from build123d import *

# Parameters (mm, degrees)
SKETCH1_W           = 38
SKETCH1_H           = 180
BOSS_EXTRUDE1_DEPTH = 25
SKETCH2_W           = 32
SKETCH2_H           = 174
CUT_EXTRUDE1_DEPTH  = 22
CHAMFER1_SIZE       = 10
FILLET1_R           = 5
FILLET2_R           = 2
SKETCH3_W           = 14
SKETCH3_H           = 10
BOSS_EXTRUDE2_DEPTH = 7
SKETCH4_W           = 14
SKETCH4_H           = 10.939467079
BOSS_EXTRUDE3_DEPTH = 7
FILLET3_R           = 3
SKETCH5_W           = 3
SKETCH5_H           = 6
CUT_EXTRUDE2_DEPTH  = 97.958754117
SKETCH6_R           = 3
CUT_EXTRUDE3_DEPTH  = 10


with BuildPart() as part:
    # Sketch1 → Boss-Extrude1 (new body)
    with BuildSketch(Plane(origin=(0, 0, 0), x_dir=(1, 0, 0), z_dir=(0, 1, 0))):
        Rectangle(SKETCH1_W, SKETCH1_H)
    extrude(amount=BOSS_EXTRUDE1_DEPTH)

    # Sketch2 → Cut-Extrude1 (cut)
    with BuildSketch(Plane.XZ):
        Rectangle(SKETCH2_W, SKETCH2_H)
    extrude(amount=-CUT_EXTRUDE1_DEPTH, mode=Mode.SUBTRACT)

    # Chamfer1
    chamfer1_edges = [part.edges().sort_by_distance(p)[0] for p in [
        (-19, 25, 0),
        (16, 22, 0),
        (0, 25, 90),
        (0, 22, -87),
        (-16, 22, 0),
        (0, 22, 87),
        (19, 25, 0),
        (0, 25, -90),
    ]]
    chamfer(chamfer1_edges, length=CHAMFER1_SIZE)

    # Fillet1
    fillet1_edges = [part.edges().sort_by_distance(p)[0] for p in [
        (19, 7.5, 90),
        (-19, 7.5, 90),
        (-19, 7.5, -90),
        (19, 7.5, -90),
    ]]
    fillet(fillet1_edges, radius=FILLET1_R)

    # Fillet2
    fillet2_edges = [part.edges().sort_by_distance(p)[0] for p in [
        (16, 6, -87),
        (-16, 6, -87),
        (-16, 6, 87),
        (16, 6, 87),
    ]]
    fillet(fillet2_edges, radius=FILLET2_R)

    # Sketch3 → Boss-Extrude2 (add)
    with BuildSketch(Plane(origin=(19, 0, 0), x_dir=(0, 0, -1), z_dir=(1, 0, 0))):
        with Locations((-75, 5)):
            Rectangle(SKETCH3_W, SKETCH3_H)
        with Locations((75, 5)):
            Rectangle(SKETCH3_W, SKETCH3_H)
    extrude(amount=BOSS_EXTRUDE2_DEPTH)

    # Sketch4 → Boss-Extrude3 (add)
    with BuildSketch(Plane.ZY.offset(19)):
        with Locations((-75, 5.469733539)):
            Rectangle(SKETCH4_W, SKETCH4_H)
        with Locations((75, 5.469733539)):
            Rectangle(SKETCH4_W, SKETCH4_H)
    extrude(amount=BOSS_EXTRUDE3_DEPTH)

    # Fillet3
    fillet3_edges = [part.edges().sort_by_distance(p)[0] for p in [
        (19, 5, 82),
        (22.5, 10, 82),
        (19, 5, 68),
        (19, 10, 75),
        (22.5, 10, 68),
        (26, 5, 82),
        (26, 5, 68),
        (26, 10, 75),
        (19, 5, -68),
        (22.5, 10, -68),
        (19, 5, -82),
        (19, 10, -75),
        (22.5, 10, -82),
        (26, 5, -68),
        (26, 5, -82),
        (26, 10, -75),
        (-19, 5.46973354, -82),
        (-22.5, 10.939467079, -82),
        (-19, 5.46973354, -68),
        (-19, 10.939467079, -75),
        (-22.5, 10.939467079, -68),
        (-26, 5.46973354, -82),
        (-26, 5.46973354, -68),
        (-26, 10.939467079, -75),
        (-19, 5.46973354, 68),
        (-22.5, 10.939467079, 68),
        (-19, 5.46973354, 82),
        (-19, 10.939467079, 75),
        (-22.5, 10.939467079, 82),
        (-26, 5.46973354, 68),
        (-26, 5.46973354, 82),
        (-26, 10.939467079, 75),
    ]]
    fillet(fillet3_edges, radius=FILLET3_R - 0.0001)  # a hair under: the kernel refuses the full size

    # Sketch5 → Cut-Extrude2 (cut, through all)
    with BuildSketch(Plane.XZ):
        with Locations((20.5, 75)):
            Rectangle(SKETCH5_W, SKETCH5_H)
        with Locations((-20.5, -75)):
            Rectangle(SKETCH5_W, SKETCH5_H)
        with Locations((20.5, -75)):
            Rectangle(SKETCH5_W, SKETCH5_H)
        with Locations((-20.5, 75)):
            Rectangle(SKETCH5_W, SKETCH5_H)
    extrude(amount=-CUT_EXTRUDE2_DEPTH, mode=Mode.SUBTRACT)

    # Sketch6 → Cut-Extrude3 (cut)
    with BuildSketch(Plane.XY.offset(90)):
        with Locations((-7, 0)):
            Circle(SKETCH6_R)
        with Locations((7, 0)):
            Circle(SKETCH6_R)
    extrude(amount=-CUT_EXTRUDE3_DEPTH, mode=Mode.SUBTRACT)


solid = part.part
Input: part model. Units: mm. Frame: model coordinates. A direction names the side the tool comes from. Coordinates: 2 decimals unless noted, no trailing zeros. Loops run counter-clockwise (first coordinate to the right, second up) from the corner with the lowest first, then second, coordinate; pieces in that order, holes last. Notation, with made-up numbers: (4, 41) -> (45, 41) arc R21 ccw to (45, 62) -> close; hole circle Ø3 at (43, -36). An arc over 180 degrees is marked (long way). Write each question's results on one line, items separated by ' | '. Start each with the question number.
Q1. Section B-B, the plane y = 4.75. State how many separate pieces and enclosed holes the cut face has, plus the area to 3 significant figures.
Q2. Reachability of faces 4 (the cylindrical face through (17, 8, 89)), 5 (the flat face through (20, 5, -72)), 6 (the cylindrical face through (-25.1, 4.03, 81.14)), 7 (the cylindrical face through (-22.51, 10.04, -68.86)), 8 (the flat face through (-16, 6, -1)) from +Z, -Z, +X, -X, +Y, -Y: full face, straight path, thin tool, end or side. Return the list, or none.
Q3. Ray query, line 1 (X direction, y = 1.25, z = 57.5); line 2 (Z direction, x = 12, y = 11.5); line 3 (Y direction, x = 3, z = 61.5). Return the intervals inside material, ascending. Write a range as from..to.
Q4. Pin query (flat end, axial travel): pin 1 (2 mm diameter, centred on x = 14.5, y = 20.5, fed in from +Z); pin 2 (1.1 mm diameter, centred on x = 22.5, y = 4.5, fed in from +Z); pin 3 (2 mm diameter, centred on x = -11, z = -42, fed in from -Y); pin 4 (8 mm diameter, centred on x = 1, y = 15.5, fed in from -Z). Return the tip coordinate at first contact, or that it passes through.
Q5. Section A-A, the plane z = -40. Return the cut outline in (x, y), plus the area to 3 significant figures.
Q6. Pull-direction query (X, two-part tool) for faces 1 (the cylindrical face through (25.1, 3.55, -68.86)), 2 (the flat face through (-26, 4, 75)), 3 (the cylindrical face through (7, 3, 89)); classes: released by +X, released by -X, zero draft, split by the parting line, or undercut.
Found:
1) separate pieces: 1 | enclosed holes: 5 | area: 1,570 mm2
2) face 4: +Z, +X, +Y, -Y | face 5: +Y, -Y | face 6: +Z, -X, +Y, -Y | face 7: -X, +Y | face 8: -Y
3) line 1: -19..-16, 16..19 | line 2: -90..-87, 87..90 | line 3: 22..25
4) pin 1: z = 85.5 | pin 2: z = 82 | pin 3: y = 16 | pin 4: z = -90
5) outline: (-19, 0) -> (-16, 0) -> (-16, 12) -> (-6, 22) -> (6, 22) -> (16, 12) -> (16, 0) -> (19, 0) -> (19, 15) -> (9, 25) -> (-9, 25) -> (-19, 15) -> close | area: 246 mm2
6) face 1: released by +X | face 2: released by -X | face 3: undercut
